For this review, take the finished solid that the model builds, in its own axes (mm). A direction names the side the tool comes from. Coordinates: 2 decimals unless noted, no trailing zeros. Use a Markdown table: item, result.
from build123d import *

# Parameters (mm, degrees)
SKETCH1_R          = 31.75
EXTRUDE1_DEPTH     = 21.082
SKETCH2_R          = 26.67
CUT_EXTRUDE1_DEPTH = 7.366
SKETCH3_R          = 26.67
CUT_EXTRUDE2_DEPTH = 7.366
SKETCH5_R          = 33.655
EXTRUDE3_DEPTH     = 2.159
CUT_EXTRUDE3_REACH = 54.967
SKETCH6_R          = 26.67
SKETCH7_R          = 33.655
EXTRUDE4_DEPTH     = 2.159
CUT_EXTRUDE4_REACH = 55.949
SKETCH8_R          = 26.67
SKETCH10_R         = 4
SKETCH10_R_2       = 1.75
CUT_EXTRUDE5_DEPTH = 54.462758337
SKETCH11_R         = 4
CUT_EXTRUDE6_DEPTH = 54.462758337
SKETCH12_R         = 4
CUT_EXTRUDE7_DEPTH = 54.462758337


with BuildPart() as part:
    # Sketch1 → Extrude1 (new body)
    with BuildSketch(Plane.XY):
        Circle(SKETCH1_R)
    extrude(amount=-EXTRUDE1_DEPTH)

    # Sketch2 → Cut-Extrude1 (cut)
    with BuildSketch(Plane.XY):
        Circle(SKETCH2_R)
    extrude(amount=-CUT_EXTRUDE1_DEPTH, mode=Mode.SUBTRACT)

    # Sketch3 → Cut-Extrude2 (cut)
    with BuildSketch(Plane(origin=(0, 0, -21.082), x_dir=(-1, 0, 0), z_dir=(0, 0, -1))):
        with Locations(Location((0, 0, 0), (0, 0, 180))):
            Circle(SKETCH3_R)
    extrude(amount=-CUT_EXTRUDE2_DEPTH, mode=Mode.SUBTRACT)

    # Sketch5 → Extrude3 (add)
    with BuildSketch(Plane.XY):
        Circle(SKETCH5_R)
    extrude(amount=EXTRUDE3_DEPTH)

    # Sketch6 → Cut-Extrude3 (cut, up to next)
    with BuildSketch(Plane.XY.offset(2.159), mode=Mode.PRIVATE) as cut_extrude3_sk1:
        with Locations(Location((0, 0, 0), (0, 0, 180))):
            Circle(SKETCH6_R)
    cut_extrude3_tool1 = extrude(cut_extrude3_sk1.sketch, amount=-CUT_EXTRUDE3_REACH, mode=Mode.PRIVATE) & part.part
    add(cut_extrude3_tool1.solids().sort_by_distance((0, 0, 2.159))[0], mode=Mode.SUBTRACT)

    # Sketch7 → Extrude4 (add)
    with BuildSketch(Plane(origin=(0, 0, -21.082), x_dir=(-1, 0, 0), z_dir=(0, 0, -1))):
        with Locations(Location((0, 0, 0), (0, 0, 180))):
            Circle(SKETCH7_R)
    extrude(amount=EXTRUDE4_DEPTH)

    # Sketch8 → Cut-Extrude4 (cut, up to next)
    with BuildSketch(Plane(origin=(0, 0, -23.241), x_dir=(-1, 0, 0), z_dir=(0, 0, -1)), mode=Mode.PRIVATE) as cut_extrude4_sk1:
        with Locations(Location((0, 0, 0), (0, 0, 180))):
            Circle(SKETCH8_R)
    cut_extrude4_tool1 = extrude(cut_extrude4_sk1.sketch, amount=-CUT_EXTRUDE4_REACH, mode=Mode.PRIVATE) & part.part
    add(cut_extrude4_tool1.solids().sort_by_distance((0, 0, -23.241))[0], mode=Mode.SUBTRACT)

    # Sweep2: sweep along a curve in space
    with BuildLine() as sweep2_path:
        ThreePointArc((33.655, 0, 2.159), (23.797678721, 23.797678721, 2.159), (0, 33.655, 2.159))
        ThreePointArc((0, 33.655, 2.159), (-23.797678721, 23.797678721, 2.159), (-33.655, 0, 2.159))
        ThreePointArc((-33.655, 0, 2.159), (-23.797678721, -23.797678721, 2.159), (0, -33.655, 2.159))
        ThreePointArc((0, -33.655, 2.159), (23.797678721, -23.797678721, 2.159), (33.655, 0, 2.159))
    # 3DSketch2 → Sweep2 (sweep)
    with BuildSketch(Plane(origin=(0, 33.655, 2.159), x_dir=(-8.931812198350224e-14, -0.9285876208505301, -0.37111323124236906), z_dir=(1, 0, 0))):
        with BuildLine():
            Line((0, 0), (0.801233466, 2.004820673))
            Line((0.801233466, 2.004820673), (2.570192884, 1.297849968))
            Line((2.570192884, 1.297849968), (10.394002025, 20.874334191))
            Line((10.394002025, 20.874334191), (8.625042607, 21.581304896))
            Line((8.625042607, 21.581304896), (9.426276074, 23.58612557))
            ThreePointArc((9.426276074, 23.58612557), (2.443828834, 12.7), (0, 0))
        make_face()
    sweep(path=sweep2_path.line)

    # Sketch10 → Cut-Extrude5 (cut, through all)
    with BuildSketch(Plane.XY.offset(-7.366)):
        Circle(SKETCH10_R)
        with Locations((0, 8)):
            Circle(SKETCH10_R_2)
        with Locations((8, 0)):
            Circle(SKETCH10_R_2)
        with Locations((0, -8)):
            Circle(SKETCH10_R_2)
        with Locations((-8, 0)):
            Circle(SKETCH10_R_2)
    extrude(amount=-CUT_EXTRUDE5_DEPTH, mode=Mode.SUBTRACT)

    # Sketch11 → Cut-Extrude6 (cut, through all)
    with BuildSketch(Plane.XY.offset(-7.366)):
        with Locations((0, 18.3)):
            Circle(SKETCH11_R)
        with Locations((18.3, 0)):
            Circle(SKETCH11_R)
        with Locations((0, -18.3)):
            Circle(SKETCH11_R)
        with Locations((-18.3, 0)):
            Circle(SKETCH11_R)
    extrude(amount=-CUT_EXTRUDE6_DEPTH, mode=Mode.SUBTRACT)

    # Sketch12 → Cut-Extrude7 (cut, through all)
    with BuildSketch(Plane.XY.offset(-7.366)):
        with Locations((12.940054096, 12.940054096)):
            Circle(SKETCH12_R)
        with Locations((12.940054096, -12.940054096)):
            Circle(SKETCH12_R)
        with Locations((-12.940054096, -12.940054096)):
            Circle(SKETCH12_R)
        with Locations((-12.940054096, 12.940054096)):
            Circle(SKETCH12_R)
    extrude(amount=-CUT_EXTRUDE7_DEPTH, mode=Mode.SUBTRACT)


solid = part.part
(1) Take a section at A-A on z = -9.5. State how many separate pieces and enclosed holes the cut face has, plus the area to 3 significant figures.
Found:
| item | result |
|---|---|
| separate pieces | 1 |
| enclosed holes | 13 |
| area | 3,600 mm^2 |
(2) For pin 1 Ø6 at (x, z) = (-26, -15) entering from -Y; pin 2 Ø1.5 at (y, z) = (-11.5, -5.5) entering from -X; pin 3 Ø1.5 at (y, z) = (-25, -18) entering from -X, all flat-tipped, find the tip position at first contact; note any pin that passes through.
Found:
| item | result |
|---|---|
| pin 1 | stops at y = -27.49 |
| pin 2 | stops at x = -34.1 |
| pin 3 | stops at x = -25.65 |
(3) For faces 3 (the face through (9.669, 0.526, -10.497)), 4 (the face through (0, 6, -13.716)), 5 (the face through (0, -6, -7.366)), list the 3-axis set-ups (+Z, -Z, +X, -X, +Y, -Y) from which the entire face can be reached by the end or side of a thin tool; tool diameter is ignored.
Found:
| item | result |
|---|---|
| face 3 | +Z, -Z |
| face 4 | -Z |
| face 5 | +Z |
(4) For line 1 along X through (y, z) = (10, -9.25); line 2 along Y through (x, z) = (0, -4.25); line 3 along X through (y, z) = (-3, -0.25), list the stretches that pass through material, from the lowest coordinate up.
Found:
| item | result |
|---|---|
| line 1 | x = -34.66 to -15.65, -10.23 to 10.23, 15.65 to 34.66 |
| line 2 | y = -35.52 to -26.67, 26.67 to 35.52 |
| line 3 | x = -34.38 to -26.5, 26.5 to 34.38 |
(5) Mouldability with a two-part tool opening along Y and no side actions: class faces 1 (the face through (15.09, -9.567, -10.497)), 2 (the face through (-20, 18, 2.159)) as pulls with the +Y half, pulls with the -Y half, needs draft (parallel to the pull), parting line crosses it, or undercut.
Found:
| item | result |
|---|---|
| face 1 | undercut |
| face 2 | needs draft |
